Could you check a few things on this model? Use its own coordinates, in mm. A direction names the side the tool comes from. Round coordinates to 2 decimals unless told otherwise and drop trailing zeros. Order: outer loops, then holes, each group sorted by start corner. A loop starts at its lowest first (then second) coordinate and runs counter-clockwise, first axis right, second up. Notation, with made-up numbers: (41, -9) - (90, -9) arc R10 cw to (90, 5) - close; hole circle Ø2 at (60, -18). An arc over 180 degrees is marked (long way). Use one line per item in the form item = value.
from build123d import *

# Parameters (mm, degrees)
SKETCH_1_R          = 4
EXTRUDE_1_DEPTH     = 17
CUT_EXTRUDE_1_DEPTH = 15


with BuildPart() as part:
    # 草图1 → 凸台-拉伸1 (new body)
    with BuildSketch(Plane(origin=(0, 0, 0), x_dir=(0, 0, -1), z_dir=(1, 0, 0))):
        Circle(SKETCH_1_R)
    extrude(amount=EXTRUDE_1_DEPTH)

    # 草图2 → 切除-拉伸1 (cut)
    with BuildSketch(Plane(origin=(17, 0, 0), x_dir=(0, 0, -1), z_dir=(1, 0, 0))):
        Polygon((-1.5, 32.646398423), (-1.5, 3.708099244), (-1.5, 2), (1.5, 2), (1.5, 3.708099244), (1.5, 32.646398423), (1.5, 90.522996781), (-1.5, 90.522996781), align=None)
    extrude(amount=-CUT_EXTRUDE_1_DEPTH, mode=Mode.SUBTRACT)


solid = part.part
Item 1: I need wall thicknesses on L1, parallel to X at y = 2.25, z = 0.5; L2, parallel to Z at x = 11, y = 3.5; L3, parallel to Z at x = 9.75, y = 2.75. Which ranges of each line are inside material? Lowest first, please.
Found:
L1 = 0 to 2
L2 = -1.94 to -1.5, 1.5 to 1.94
L3 = -2.9 to -1.5, 1.5 to 2.9
Item 2: Imagine slicing it at D-D on z = -3.5. Please give me the cut outline in (x, y).
Found:
outline = (0, -1.94) - (17, -1.94) - (17, 1.94) - (0, 1.94) - close
Item 3: Imagine slicing it at C-C on x = 11.25. Please give me the cut outline in (y, z), plus the area to 3 significant figures.
Found:
outline = (2, -1.5) - (2, 1.5) - (3.71, 1.5) arc R4 ccw (long way) to (3.71, -1.5) - close
area = 44.6 mm2
Item 4: Imagine slicing it at B-B on y = 3.5. Please give me the cut outline in (x, z), plus the area to 3 significant figures.
Found:
outline = (0, -1.94) - (17, -1.94) - (17, -1.5) - (2, -1.5) - (2, 1.5) - (17, 1.5) - (17, 1.94) - (0, 1.94) - close
area = 20.8 mm2
Item 5: If we mould it in two halves opening along Z, with no side actions, what happens to faces 1 (the face through (8.381, -3.905, 0.867)), 2 (the face through (0, 0, 0)), 3 (the face through (10, 3, 1.5)), 4 (the face through (10, 2, 0))? For each: released by +Z, released by -Z, zero draft, split by the parting line, or undercut.
Found:
face_1 = split by the parting line
face_2 = zero draft
face_3 = undercut
face_4 = undercut
Item 6: For faces 5 (the face through (2, 3, 0)), 6 (the face through (17, 0, 0)), which set-ups out of +Z, -Z, +X, -X, +Y, -Y let a thin tool reach every point of the face, with its end or its side?
Found:
face_5 = +X, +Y
face_6 = +Z, -Z, +X, +Y, -Y
Item 7: Imagine slicing it at A-A on z = 0. Please give me the cut outline in (x, y), plus the area to 3 significant figures.
Found:
outline = (0, -4) - (17, -4) - (17, 2) - (2, 2) - (2, 4) - (0, 4) - close
area = 106 mm2
Item 8: Will these pins go through, and if not, where does the flat tip stop? P1, Ø1.9, axis at x = 11, y = 3, coming from the -Z side; P2, Ø1.5, axis at x = 6, z = 0.5, coming from the +Y side; P3, Ø1.5, axis at x = 2, y = 1, coming from the -Z side; P4, Ø3, axis at x = 9.5, z = 1, coming from the -Y side.
Found:
P1 = -3.43
P2 = 2
P3 = -3.99
P4 = -4
